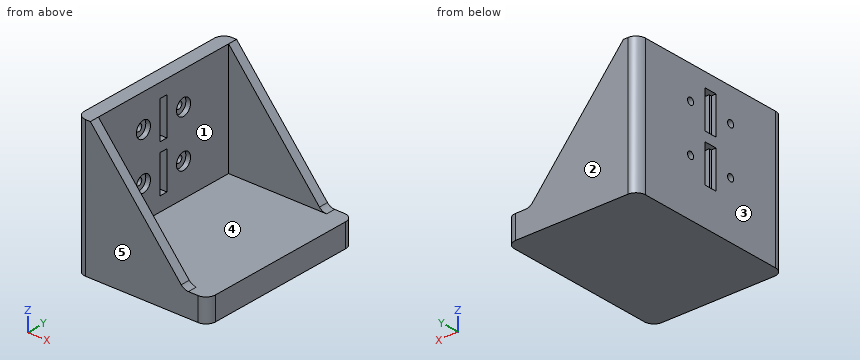
from build123d import *

# Parameters (mm, degrees)
F0_W      = 56
F0_H      = 73
F1_DEPTH  = 10
F2_W      = 40
F2_H      = 4
F3_DEPTH  = 48
F5_DEPTH  = 73.001
F6_R      = 4
F7_W      = 1.035
F7_H      = 16
F8_DEPTH  = 2
F7_W_2    = 3.45
F9_DEPTH  = 6
F10_R     = 3.5
F10_R_2   = 1.5
F11_DEPTH = 2
F12_DEPTH = 6


with BuildPart() as f1:
    # F0 (on Top) → F1 (new body)
    with BuildSketch(Plane.XY):
        with Locations((28, 36.5)):
            Rectangle(F0_W, F0_H)
    extrude(amount=F1_DEPTH)

    # F2 (on face) → F3 (join)
    with BuildSketch(Plane.XY.offset(10)):
        Polygon((6, 73), (0, 73), (0, 0), (6, 0), (6, 4), (6, 69), align=None)
        with Locations((26, 71)):
            Rectangle(F2_W, F2_H)
        with Locations((26, 2)):
            Rectangle(F2_W, F2_H)
    extrude(amount=F3_DEPTH)

    # F4 (on face) → F5 (cut, through all)
    with BuildSketch(Plane.XZ):
        Polygon((6, 58), (46, 10), (46, 58), align=None)
    extrude(amount=-F5_DEPTH, mode=Mode.SUBTRACT)

    # F6
    f6_edges = [f1.edges().sort_by_distance(p)[0] for p in [
        (0, 0, 29),
        (56, 0, 5),
        (46, 2, 10),
        (46, 71, 10),
        (56, 73, 5),
        (0, 73, 29),
    ]]
    fillet(f6_edges, radius=F6_R)

    # F7 (on face) → F8 (cut)
    with BuildSketch(Plane(origin=(0, 0, 0), x_dir=(0, -1, 0), z_dir=(-1, 0, 0))):
        with Locations((-38.7425, 44)):
            Rectangle(F7_W, F7_H)
        with Locations((-34.2575, 44)):
            Rectangle(F7_W, F7_H)
        with Locations((-34.2575, 24)):
            Rectangle(F7_W, F7_H)
        with Locations((-38.7425, 24)):
            Rectangle(F7_W, F7_H)
    extrude(amount=-F8_DEPTH, mode=Mode.SUBTRACT)

    # F7 (on face) → F9 (cut, through all)
    with BuildSketch(Plane(origin=(0, 0, 0), x_dir=(0, -1, 0), z_dir=(-1, 0, 0))):
        with Locations((-36.5, 44)):
            Rectangle(F7_W_2, F7_H)
        with Locations((-36.5, 24)):
            Rectangle(F7_W_2, F7_H)
    extrude(amount=-F9_DEPTH, mode=Mode.SUBTRACT)

    # F10 (on face) → F11 (cut)
    with BuildSketch(Plane.YZ.offset(6)):
        with Locations((26.5, 44)):
            Circle(F10_R)
        with Locations((26.5, 44)):
            Circle(F10_R_2, mode=Mode.SUBTRACT)
        with Locations((46.5, 44)):
            Circle(F10_R)
        with Locations((46.5, 44)):
            Circle(F10_R_2, mode=Mode.SUBTRACT)
        with Locations((46.5, 24)):
            Circle(F10_R)
        with Locations((46.5, 24)):
            Circle(F10_R_2, mode=Mode.SUBTRACT)
        with Locations((26.5, 24)):
            Circle(F10_R)
        with Locations((26.5, 24)):
            Circle(F10_R_2, mode=Mode.SUBTRACT)
    extrude(amount=-F11_DEPTH, mode=Mode.SUBTRACT)

    # F10 (on face) → F12 (cut, through all)
    with BuildSketch(Plane.YZ.offset(6)):
        with Locations((26.5, 44)):
            Circle(F10_R_2)
        with Locations((46.5, 44)):
            Circle(F10_R_2)
        with Locations((46.5, 24)):
            Circle(F10_R_2)
        with Locations((26.5, 24)):
            Circle(F10_R_2)
    extrude(amount=-F12_DEPTH, mode=Mode.SUBTRACT)


solid = f1.part
Input: part model. Units: mm. Frame: model coordinates. Face numbers are marked on the shaded views. A direction names the side the tool comes from. Give positions to 0.01 mm unless a question says otherwise; leave off trailing zeros. Write each loop counter-clockwise with the first axis right and the second up, starting at its lowest first coordinate (ties: lowest second). Pieces come first, ordered by that corner, then holes. Notation, with made-up numbers: M 27,-5 L 34,-5 A34 ccw 34,29 Z; hole C 58,61.25 d7. An arc over 180 degrees is marked long. Use one line per item in the form item = value.
1. Cut plane C-C on x = 18. Return loops of the section in (y, z).
Outcome:
outline = M 0,0 L 73,0 L 73,43.6 L 69,43.6 L 69,10 L 4,10 L 4,43.6 L 0,43.6 Z
2. Mould query, pull axis Y, two halves, no side actions, for the marked faces 1, 2 and 3. Classes: released by +Y, released by -Y, zero draft, split by the parting line, or undercut.
Outcome:
face_1 = undercut
face_2 = released by +Y
face_3 = zero draft
3. First-contact query: P1, Ø6.5, axis at y = 26.5, z = 44, coming from the +X side; P2, Ø5, axis at x = 31.5, y = 8, coming from the +Z side; P3, Ø1.5, axis at x = 42.5, z = 16.5, coming from the +Y side; P4, Ø1.6, axis at x = 1, z = 21.5, coming from the -Y side. Flat tips, straight axial feed; report the tip coordinate or a pass-through.
Outcome:
P1 = 4
P2 = 10
P3 = through
P4 = 0.66
4. Cut plane D-D on z = 44. State how many separate pieces and enclosed holes the cut face has, and give its area (3 significant figures).
Outcome:
separate_pieces = 4
enclosed_holes = 0
area = 448 mm²
5. Reachability of the marked faces 4 and 5 from +Z, -Z, +X, -X, +Y, -Y: full face, straight path, thin tool, end or side. Return the list, or none.
Outcome:
face_4 = +Z, +X
face_5 = +Z, -Z, +X, -X, -Y
6. Ray query, L1, parallel to Z at x = 5, y = 46.5; L2, parallel to Z at x = 3.25, y = 26.5; L3, parallel to Y at x = 11.5, z = 29. Return the intervals inside material, ascending.
Outcome:
L1 = 0 to 20.5, 27.5 to 40.5, 47.5 to 58
L2 = 0 to 22.5, 25.5 to 42.5, 45.5 to 58
L3 = 0 to 4, 69 to 73
7. Cut plane A-A on z = 50.5. Return loops of the section in (x, y) (3 decimals).
Outcome:
outline = M 0,4 A4 ccw 4,0 L 12.25,0 L 12.25,4 L 6,4 L 6,34.775 L 2,34.775 L 2,33.74 L 0,33.74 Z; M 0,39.26 L 2,39.26 L 2,38.225 L 6,38.225 L 6,69 L 12.25,69 L 12.25,73 L 4,73 A4 ccw 0,69 Z
8. Cut plane B-B on y = 26.5. Return loops of the section in (x, z), and give its area (3 significant figures).
Outcome:
outline = M 0,0 L 56,0 L 56,10 L 6,10 L 6,20.5 L 4,20.5 L 4,22.5 L 0,22.5 Z; M 0,25.5 L 4,25.5 L 4,27.5 L 6,27.5 L 6,40.5 L 4,40.5 L 4,42.5 L 0,42.5 Z; M 0,45.5 L 4,45.5 L 4,47.5 L 6,47.5 L 6,58 L 0,58 Z
area = 796 mm²
